Can you work these out from the model? Positions are in its coordinate system, mm. A direction names the side the tool comes from. Round coordinates to 2 decimals unless told otherwise and drop trailing zeros. Loops run counter-clockwise (first coordinate to the right, second up) from the corner with the lowest first, then second, coordinate; pieces in that order, holes last. Notation, with made-up numbers: M 18.5,40 L 30.5,40 A22 ccw 30.5,46 Z; hole C 36,64 d8. An arc over 180 degrees is marked long. Return JSON: item names as keys, results as strings.
```python
from build123d import *

# Parameters (mm, degrees)
F0_W     = 85.4783095419
F0_H     = 59.5757905394
F1_DEPTH = 50.8
F2_W     = 28.3403936774
F2_H     = 12.6175824553
F2_R     = 2.3774170248
F2_W_2   = 25.0316578895
F2_H_2   = 13.0906309932
F2_R_2   = 2.2246950569
F2_W_3   = 70.6177633256
F2_H_3   = 11.6556163412
F3_DEPTH = 0.254
F4_SIZE  = 5.08
F5_R     = 5.08
F6_SCALE = 0.5
F7_R     = 2.413
F8_DEPTH = 10.16


with BuildPart() as f1:
    # F0 (on Front) → F1 (new body)
    with BuildSketch(Plane.XZ):
        with Locations((6.331725046, 10.3610074148)):
            Rectangle(F0_W, F0_H)
    extrude(amount=F1_DEPTH)

    # F2 (on face) → F3 (join)
    with BuildSketch(Plane.XZ.offset(50.8)):
        with Locations((-14.1701968387, 22.8276690468)):
            Rectangle(F2_W, F2_H)
        with Locations((-15.9050039947, 23.1631565839)):
            Circle(F2_R, mode=Mode.SUBTRACT)
        with Locations((22.638711147, 22.3876358941)):
            Rectangle(F2_W_2, F2_H_2)
        with Locations((23.0593848974, 22.195097059)):
            Circle(F2_R_2, mode=Mode.SUBTRACT)
        Polygon((9.9397739728, 7.435437333), (9.9397739728, 10.3037140541), (8.3890665016, 12.7166619788), (5.7799902246, 13.9081871902), (2.9409084248, 13.4999888525), (0.7732095137, 11.6216670538), (-0.0348774207, 8.8695756935), (0.7732095137, 6.1174843332), (2.9409084248, 4.2391625345), (5.7799902246, 3.8309641968), (8.3890665016, 5.0224894082), align=None)
        with Locations((6.9684879854, -5.284418934)):
            Rectangle(F2_W_3, F2_H_3)
    extrude(amount=F3_DEPTH)

    # F4
    f4_edges = [f1.edges().sort_by_distance(p)[0] for p in [
        (49.07088, -25.4, 40.148903),
        (-36.40743, -25.4, 40.148903),
        (6.331725, 0, 40.148903),
        (6.331725, -50.8, 40.148903),
        (-36.40743, -25.4, -19.426888),
        (49.07088, -25.4, -19.426888),
        (6.331725, 0, -19.426888),
        (6.331725, -50.8, -19.426888),
    ]]
    chamfer(f4_edges, length=F4_SIZE)

    # F5
    f5_edges = [f1.edges().sort_by_distance(p)[0] for p in [
        (-36.40743, -50.8, 10.361007),
        (49.07088, -50.8, 10.361007),
    ]]
    fillet(f5_edges, radius=F5_R)


with BuildPart() as f1_1:
    # F6: moved
    add(f1.part.scale(F6_SCALE))

    # F7 (on face) → F8 (join)
    with BuildSketch(Plane(origin=(0, 0, -9.7134439275), x_dir=(1, 0, 0), z_dir=(0, 0, -1))):
        with Locations((3.165862523, 12.7)):
            Circle(F7_R)
    extrude(amount=F8_DEPTH)


solid = f1_1.part
```
Q1. Suppose I cut it at C-C, the plane y = -5.75. Please give me the cut outline in (x, z), plus the area to 3 significant figures.
Results:
{"outline": "M -18.2,-7.17 L -15.66,-9.71 L 22,-9.71 L 24.54,-7.17 L 24.54,17.53 L 22,20.07 L -15.66,20.07 L -18.2,17.53 Z", "area": "1,260 mm2"}
Q2. Thinking about a two-plate mould opening in Z: for faces 3 (the flat face through (12, -25.4, 11)), 4 (the flat face through (-16.916, -12.155, -8.461)), 5 (the cylindrical face through (-17.479, -24.636, 5.364)), 6 (the flat face through (-8, -25.4, 12)), which applies, pulls with the +Z half, pulls with the -Z half, needs draft (parallel to the pull), parting line crosses it, or undercut?
Results:
{"face 3": "undercut", "face 4": "pulls with the -Z half", "face 5": "needs draft", "face 6": "undercut"}
Q3. If I drill on line 1 along Z through (x, y) = (9, -4); line 2 along Y through (x, z) = (4, 13); line 3 along Z through (x, y) = (1.5, -2.5), over which ranges is the centre line in solid material (lowest first)?
Results:
{"line 1": "z = -9.71 to 20.07", "line 2": "y = -25.4 to 0", "line 3": "z = -9.67 to 20.03"}
Q4. Suppose I cut it at A-A, the plane y = -12.7. Please give me the cut outline in (x, z), plus the area to 3 significant figures.
Results:
{"outline": "M -18.2,-7.17 L -15.66,-9.71 L 0.75,-9.71 L 0.75,-19.87 L 5.58,-19.87 L 5.58,-9.71 L 22,-9.71 L 24.54,-7.17 L 24.54,17.53 L 22,20.07 L -15.66,20.07 L -18.2,17.53 Z", "area": "1,310 mm2"}
Q5. Suppose I cut it at D-D, the plane x = 8.5. Please give me the cut outline in (y, z), plus the area to 3 significant figures.
Results:
{"outline": "M -25.53,-5.56 L -25.4,-5.56 L -25.4,-7.17 L -22.86,-9.71 L -2.54,-9.71 L 0,-7.17 L 0,17.53 L -2.54,20.07 L -22.86,20.07 L -25.4,17.53 L -25.4,14.47 L -25.53,14.47 L -25.53,7.92 L -25.4,7.92 L -25.4,0.27 L -25.53,0.27 Z", "area": "745 mm2"}
Q6. I'm going to push a flat-ended pin straight in: pin 1 Ø4 at (x, y) = (-2, -22.5) entering from -Z. Where does the tip first touch, or does it pass through?
Results:
{"pin 1": "stops at z = -9.71"}
Q7. On a 3-axis mill with a long thin cutter (end or side, diameter ignored), from which of +Z, -Z, +X, -X, +Y, -Y can I reach the whole of each face in a straight line? I mean faces 1 (the cylindrical face through (4.28, -10.56, -14.72)), 2 (the flat face through (3, -13, 20.074)). Say none if no direction works.
Results:
{"face 1": "-Z", "face 2": "+Z, +X, -X, +Y, -Y"}
Q8. Suppose I cut it at B-B, the plane x = -10. Please give me the cut outline in (y, z), plus the area to 3 significant figures.
Results:
{"outline": "M -25.53,-5.56 L -25.4,-5.56 L -25.4,-7.17 L -22.86,-9.71 L -2.54,-9.71 L 0,-7.17 L 0,17.53 L -2.54,20.07 L -22.86,20.07 L -25.4,17.53 L -25.4,14.57 L -25.53,14.57 L -25.53,8.26 L -25.4,8.26 L -25.4,0.27 L -25.53,0.27 Z", "area": "745 mm2"}
